Geometry: final body of the model. Coordinates: model frame, mm. Face numbers are marked on the shaded views. A direction names the side the tool comes from. Coordinates: 2 decimals unless noted, no trailing zeros. Write each loop counter-clockwise with the first axis right and the second up, starting at its lowest first coordinate (ties: lowest second). Pieces come first, ordered by that corner, then holes.
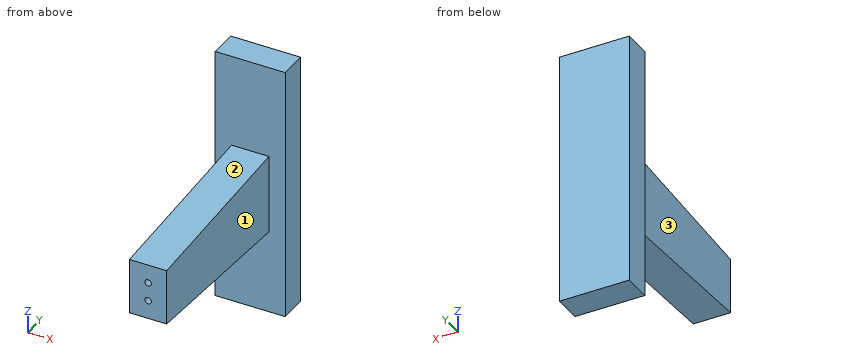
from build123d import *

# Parameters (mm, degrees)
BOSS_EXTRUDE1_DEPTH = 40
BOSS_EXTRUDE2_START = -17.5
SKETCH2_W           = 275
SKETCH2_H           = 30
BOSS_EXTRUDE2_DEPTH = 75
SKETCH4_R           = 3.5
CUT_EXTRUDE1_DEPTH  = 10


with BuildPart() as part:
    # Sketch1 → Boss-Extrude1 (new body)
    with BuildSketch(Plane(origin=(0, 0, 0), x_dir=(0, 0, -1), z_dir=(1, 0, 0))):
        Polygon((-30, 0), (30, 0), (42.5, 200), (132.5, 200), (132.5, 230), (-142.5, 230), (-142.5, 200), (-42.5, 200), align=None)
    extrude(amount=BOSS_EXTRUDE1_DEPTH)

    # Sketch2 → Boss-Extrude2 (add)
    with BuildSketch(Plane(origin=(0, 0, 0), x_dir=(0, 0, -1), z_dir=(1, 0, 0)).offset(BOSS_EXTRUDE2_START)):
        with Locations((-5, 215)):
            Rectangle(SKETCH2_W, SKETCH2_H)
    extrude(amount=BOSS_EXTRUDE2_DEPTH)

    # Sketch4 → Cut-Extrude1 (cut)
    with BuildSketch(Plane(origin=(0, 0, 0), x_dir=(1, 0, 0), z_dir=(0, 1, 0))):
        with Locations(Location((20, -10, 0), (0, 0, 270))):
            Circle(SKETCH4_R)
        with Locations(Location((20, 10, 0), (0, 0, 270))):
            Circle(SKETCH4_R)
    extrude(amount=CUT_EXTRUDE1_DEPTH, mode=Mode.SUBTRACT)


solid = part.part
Item 1: Set-up query: the marked faces 1, 2 and 3. Return all of +Z, -Z, +X, -X, +Y, -Y with unobstructed straight access to the full face (end or side cutting, diameter ignored); none if empty.
Derived:
face 1: +Z, -Z, +X, -Y
face 2: +Z, +X, -X, -Y
face 3: +Z, -Z, -X, -Y
Item 2: Pin query (flat end, axial travel): pin 1 (1 mm diameter, centred on y = 79.5, z = -7.5, fed in from -X); pin 2 (2 mm diameter, centred on x = 18.5, z = 11.5, fed in from -Y); pin 3 (7.5 mm diameter, centred on x = 21, z = -9.5, fed in from -Y); pin 4 (1 mm diameter, centred on y = 97, z = -30, fed in from +X). Return the tip coordinate at first contact, or that it passes through.
Derived:
pin 1: stops at x = 0
pin 2: stops at y = 10
pin 3: stops at y = 0
pin 4: stops at x = 40
Item 3: Section B-B, the plane z = 10. Output: boundary loops of the cut face in (x, y), plus the area to 3 significant figures.
Derived:
outline: (-17.5, 200) - (0, 200) - (0, 0) - (16.5, 0) - (16.5, 10) - (23.5, 10) - (23.5, 0) - (40, 0) - (40, 200) - (57.5, 200) - (57.5, 230) - (-17.5, 230) - close
area: 10,200 mm2
Item 4: Section A-A, the plane x = 20. Output: boundary loops of the cut face in (y, z), plus the area to 3 significant figures.
Derived:
outline: (0, -30) - (200, -42.5) - (200, -132.5) - (230, -132.5) - (230, 142.5) - (200, 142.5) - (200, 42.5) - (0, 30) - (0, 13.5) - (10, 13.5) - (10, 6.5) - (0, 6.5) - (0, -6.5) - (10, -6.5) - (10, -13.5) - (0, -13.5) - close
area: 22,600 mm2
Item 5: Section D-D, the plane z = 76. Output: boundary loops of the cut face in (x, y), plus the area to 3 significant figures.
Derived:
outline: (-17.5, 200) - (57.5, 200) - (57.5, 230) - (-17.5, 230) - close
area: 2,250 mm2
Item 6: Section C-C, the plane y = 68. Output: boundary loops of the cut face in (x, z), plus the area to 3 significant figures.
Derived:
outline: (0, -34.25) - (40, -34.25) - (40, 34.25) - (0, 34.25) - close
area: 2,740 mm2
Item 7: Material intervals for probe 1 along X at (y, z) = (7.5, 10); probe 2 along Y at (x, z) = (35, 47); probe 3 along X at (y, z) = (117.5, 1), sorted ascending.
Derived:
probe 1: x = 0 to 16.5, 23.5 to 40
probe 2: y = 200 to 230
probe 3: x = 0 to 40
